```python
from build123d import *

# Parameters (mm, degrees)
F1_DEPTH = 12.7
F2_D     = 19.44624


with BuildPart() as f1:
    # F0 (on Front) → F1 (new body)
    with BuildSketch(Plane.XZ):
        with BuildLine():
            Line((-8.9467406929, 65.1259068947), (-59.7467406929, 65.1259068947))
            ThreePointArc((-59.7467406929, 65.1259068947), (-77.707252935, 57.6864191368), (-85.1467406929, 39.7259068947))
            Line((-85.1467406929, 39.7259068947), (-85.1467406929, -49.1740931053))
            ThreePointArc((-85.1467406929, -49.1740931053), (-81.4269968139, -58.1543492264), (-72.4467406929, -61.8740931053))
            Line((-72.4467406929, -61.8740931053), (-67.6969406929, -61.8740931053))
            Line((-67.6969406929, -61.8740931053), (-67.6969406929, -67.2842931053))
            ThreePointArc((-67.6969406929, -67.2842931053), (-66.9529919171, -69.0803443295), (-65.1569406929, -69.8242931053))
            Line((-65.1569406929, -69.8242931053), (-3.5365406929, -69.8242931053))
            ThreePointArc((-3.5365406929, -69.8242931053), (-1.7404894686, -69.0803443295), (-0.9965406929, -67.2842931053))
            Line((-0.9965406929, -67.2842931053), (-0.9965406929, -61.8740931053))
            Line((-0.9965406929, -61.8740931053), (3.7532593071, -61.8740931053))
            ThreePointArc((3.7532593071, -61.8740931053), (12.7335154282, -58.1543492264), (16.4532593071, -49.1740931053))
            Line((16.4532593071, -49.1740931053), (16.4532593071, 39.7259068947))
            ThreePointArc((16.4532593071, 39.7259068947), (9.0137715493, 57.6864191368), (-8.9467406929, 65.1259068947))
        make_face()
    extrude(amount=F1_DEPTH)

    # F2 (through all)
    with Locations(Plane(origin=(0, 0, 0), x_dir=(1, 0, 0), z_dir=(0, 1, 0))):
        with Locations((-34.3467406929, -32.2189068947)):
            Hole(F2_D / 2)


solid = f1.part
```
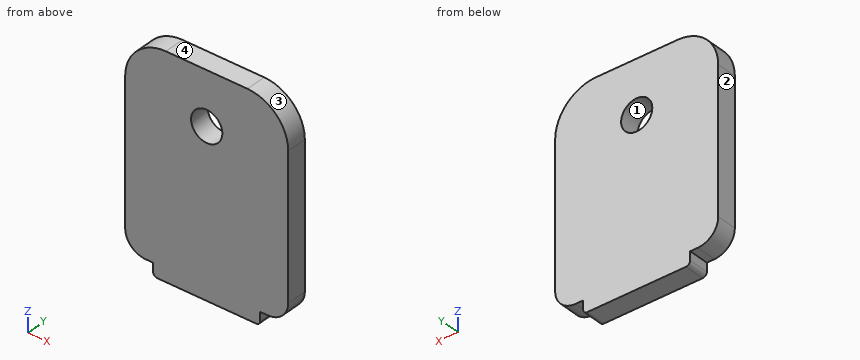
Read the model definition and answer for the solid it produces. Units are mm, in the model's axes. Face numbers are marked on the shaded views. Give positions to 0.01 mm unless a question says otherwise; leave off trailing zeros. Loops run counter-clockwise (first coordinate to the right, second up) from the corner with the lowest first, then second, coordinate; pieces in that order, holes last.
Item 1: The part is cut by section C-C (y = -3). Write down the section's boundary in (x, z).
Item 2: The part is cut by section A-A (z = 34). Write down the section's boundary in (x, y), and give its area (3 significant figures).
Item 3: The part is cut by section D-D (z = 48). Write down the section's boundary in (x, y), and give its area (3 significant figures).
Item 4: Each of these flat-tipped pins is pushed along its axis until it touches: pin 1 Ø5 at (x, y) = (0.5, -6.5) entering from -Z; pin 2 Ø4 at (x, y) = (-4.5, -6) entering from +Z; pin 3 Ø1.6 at (y, z) = (-8.5, -65) entering from +X; pin 4 Ø15.5 at (x, z) = (-34.35, 32.22) entering from +Y. Where does it stop, or does it pass through?
Item 5: Find the intervals of material crossed by line 1 along Z through (x, y) = (-42.5, -6.25); line 2 along Z through (x, y) = (-35, -2.5); line 3 along X through (y, z) = (-10.75, 38.5), in increasing order.
Item 6: The part is cut by section B-B (x = -34). Write down the section's boundary in (y, z), and give its area (3 significant figures).
Item 7: The mould has two halves that part along X. Classify the marked faces 1, 2, 3 and 4: released by +X, released by -X, zero draft, split by the parting line, or undercut.
Taken from the geometry:
1. outline: (-85.15, -49.17) arc R12.7 ccw to (-72.45, -61.87) - (-67.7, -61.87) - (-67.7, -67.28) arc R2.54 ccw to (-65.16, -69.82) - (-3.54, -69.82) arc R2.54 ccw to (-1, -67.28) - (-1, -61.87) - (3.75, -61.87) arc R12.7 ccw to (16.45, -49.17) - (16.45, 39.73) arc R25.4 ccw to (-8.95, 65.13) - (-59.75, 65.13) arc R25.4 ccw to (-85.15, 39.73) - close; hole circle Ø19.45 at (-34.35, 32.22)
2. outline: (-85.15, -12.7) - (-43.91, -12.7) - (-43.91, 0) - (-85.15, 0) - close; (-24.79, -12.7) - (16.45, -12.7) - (16.45, 0) - (-24.79, 0) - close
2. area: 1,050 mm2
3. outline: (-83.76, -12.7) - (15.07, -12.7) - (15.07, 0) - (-83.76, 0) - close
3. area: 1,260 mm2
4. pin 1: stops at z = -69.31
4. pin 2: stops at z = 65.01
4. pin 3: stops at x = -1
4. pin 4: passes through
5. line 1: z = -69.82 to 26.92, 37.52 to 65.13
5. line 2: z = -69.82 to 22.52, 41.92 to 65.13
5. line 3: x = -85.15 to -41.77, -26.92 to 16.45
6. outline: (-12.7, -69.82) - (0, -69.82) - (0, 22.5) - (-12.7, 22.5) - close; (-12.7, 41.94) - (0, 41.94) - (0, 65.13) - (-12.7, 65.13) - close
6. area: 1,470 mm2
7. face 1: undercut
7. face 2: released by -X
7. face 3: released by +X
7. face 4: zero draft
